Work out the finished part from the listing and answer in its coordinate system (mm). Round coordinates to 2 decimals unless told otherwise and drop trailing zeros. Order: outer loops, then holes, each group sorted by start corner. A loop starts at its lowest first (then second) coordinate and runs counter-clockwise, first axis right, second up. Notation, with made-up numbers: (-34.5, 83.25) - (0.5, 83.25) arc R26 ccw to (0.5, 115.25) - close; hole circle Ø2 at (-12, -12). An arc over 180 degrees is marked (long way). Use one line per item in the form item = value. Start each with the question number.
Q1. The part is cut by section C-C on z = 1.45. Determine the outline of the cut face in (x, y).
Q2. For a pull along Y with two mould halves and no side action, classify faces 1 (the flat face through (0, 0, 4)), 2 (the cylindrical face through (-12.248, 0.099, 1.972)), 3 (the cylindrical face through (7.752, 0.099, 1.972)), 4 (the flat face through (0, -4.5, 2)) as +Y half, -Y half, draft (parallel to the pull), parting line (faces both ways), or undercut.
Q3. The part is cut by section D-D on x = 11.75. Determine the outline of the cut face in (y, z).
Q4. The part is cut by section A-A on y = 0. Determine the outline of the cut face in (x, z).
Q5. The part is cut by section B-B on x = -11.25. Determine the outline of the cut face in (y, z).
Q6. Find the intervals of material crossed by line 1 (X direction, y = 1.5, z = 0.75); line 2 (X direction, y = 1.25, z = 2.4); line 3 (Y direction, x = -10, z = 1.2), in increasing order. Write a range as [from, to].
from build123d import *

# Parameters (mm, degrees)
SKETCH1_R           = 4.5
SKETCH1_R_2         = 2.25
BOSS_EXTRUDE1_DEPTH = 4


with BuildPart() as part:
    # Sketch1 → Boss-Extrude1 (new body)
    with BuildSketch(Plane.XY):
        with Locations((-10, 0)):
            Circle(SKETCH1_R)
        with Locations((-10, 0)):
            Circle(SKETCH1_R_2, mode=Mode.SUBTRACT)
        with BuildLine():
            Line((10, 4.5), (-10, 4.5))
            ThreePointArc((-10, 4.5), (-6.818019485, 3.181980515), (-5.5, 0))
            ThreePointArc((-5.5, 0), (-6.818019485, -3.181980515), (-10, -4.5))
            Line((-10, -4.5), (10, -4.5))
            ThreePointArc((10, -4.5), (5.5, 0), (10, 4.5))
        make_face()
        with Locations((10, 0)):
            Circle(SKETCH1_R)
        with Locations((10, 0)):
            Circle(SKETCH1_R_2, mode=Mode.SUBTRACT)
    extrude(amount=BOSS_EXTRUDE1_DEPTH)


solid = part.part
Found:
q1.outline = (-10, -4.5) - (10, -4.5) arc R4.5 ccw to (10, 4.5) - (-10, 4.5) arc R4.5 ccw to start; hole circle Ø4.5 at (-10, 0); hole circle Ø4.5 at (10, 0)
q2.face_1 = draft
q2.face_2 = undercut
q2.face_3 = undercut
q2.face_4 = -Y half
q3.outline = (-4.15, 0) - (-1.41, 0) - (-1.41, 4) - (-4.15, 4) - close; (1.41, 0) - (4.15, 0) - (4.15, 4) - (1.41, 4) - close
q4.outline = (-14.5, 0) - (-12.25, 0) - (-12.25, 4) - (-14.5, 4) - close; (-7.75, 0) - (7.75, 0) - (7.75, 4) - (-7.75, 4) - close; (12.25, 0) - (14.5, 0) - (14.5, 4) - (12.25, 4) - close
q5.outline = (-4.32, 0) - (-1.87, 0) - (-1.87, 4) - (-4.32, 4) - close; (1.87, 0) - (4.32, 0) - (4.32, 4) - (1.87, 4) - close
q6.line_1 = [-14.24, -11.68], [-8.32, 8.32], [11.68, 14.24]
q6.line_2 = [-14.32, -11.87], [-8.13, 8.13], [11.87, 14.32]
q6.line_3 = [-4.5, -2.25], [2.25, 4.5]
